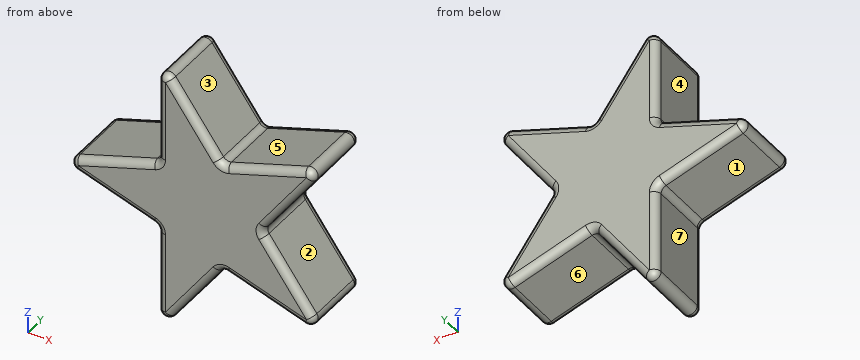
```python
from build123d import *

# Parameters (mm, degrees)
F1_DEPTH = 50.8
F2_F1_R  = 5.08
F2_F2_R  = 5.08


with BuildPart() as f1:
    # F0 (on Front) → F1 (new body)
    with BuildSketch(Plane.XZ):
        Polygon((44.7892362247, -61.6470949714), (0, 0), (44.7892362247, 61.6470949714), (-27.681270317, 38.1), (-72.4705065417, 99.7470949714), (-72.4705065417, 23.5470949714), (-144.9410130834, 0), (-72.4705065417, -23.5470949714), (-72.4705065417, -99.7470949714), (-27.681270317, -38.1), align=None)
    extrude(amount=-F1_DEPTH)

    # F2: fillet of radius 5.08 on 21 edges, made by hand

    # F2_f1
    f2_f1_edges = [f1.edges().sort_by_distance(p)[0] for p in [
        (-27.681270317, 25.4, -38.1),
        (-72.4705065417, 25.4, -23.5470949714),
        (-72.4705065417, 25.4, 23.5470949714),
        (-27.681270317, 25.4, 38.1),
        (0, 25.4, 0),
    ]]
    fillet(f2_f1_edges, radius=F2_F1_R)

    # F2_f2
    f2_f2_edges = [f1.edges().sort_by_distance(p)[0] for p in [
        (-72.4705065417, 25.4, 99.7470949714),
        (-144.9410130834, 25.4, 0),
        (44.7892362247, 25.4, 61.6470949714),
        (44.7892362247, 25.4, -61.6470949714),
        (-72.4705065417, 25.4, -99.7470949714),
        (-72.4705065417, 50.8, -63.4925129925),
        (-51.1605979265, 50.8, -70.4165220265),
        (10.3090797881, 50.8, -50.4438130159),
        (-110.4608566468, 50.8, 11.2032819554),
        (-51.1605979265, 50.8, 70.4165220265),
        (23.4793276095, 50.8, 32.3165220265),
        (23.4793276095, 0, 32.3165220265),
        (10.3090797881, 0, 50.4438130159),
        (-72.4705065417, 0, 63.4925129925),
        (-110.4608566468, 0, -11.2032819554),
        (-51.1605979265, 0, -70.4165220265),
        (-27.3106893113, 0, -39.2405310605),
        (-73.4407002103, 0, -24.251981932),
        (-73.4407002103, 0, 24.251981932),
        (-27.3106893113, 0, 39.2405310605),
        (1.1992253257, 0, 0),
        (1.1992253257, 50.8, 0),
        (-27.3106893113, 50.8, 39.2405310605),
        (-73.4407002103, 50.8, 24.251981932),
        (-27.3106893113, 50.8, -39.2405310605),
        (-73.4407002103, 50.8, -24.251981932),
    ]]
    fillet(f2_f2_edges, radius=F2_F2_R)


solid = f1.part
```
The listing builds one solid part. Answer for the finished solid, in the listing's coordinates (mm). Face numbers are marked on the shaded views. A direction names the side the tool comes from. Give positions to 0.01 mm unless a question says otherwise; leave off trailing zeros. Loops run counter-clockwise (first coordinate to the right, second up) from the corner with the lowest first, then second, coordinate; pieces in that order, holes last. Notation, with made-up numbers: (-25, 50.5) - (-13, 50.5) arc R14 ccw to (-13, 74.5) - close; hole circle Ø3 at (-39, 8). An arc over 180 degrees is marked (long way). Return JSON: item names as keys, results as strings. Group by question number.
1. Given pin 1 Ø1 at (y, z) = (38, -60) entering from -X; pin 2 Ø3 at (x, y) = (-100.5, 35.5) entering from -Z; pin 3 Ø4 at (x, y) = (-86, 30) entering from +Z, each flat-ended and moving along its own axis, determine where each tip first touches the part or whether it passes through.
2. Which of the six approach directions +Z, -Z, +X, -X, +Y, -Y give full straight-line access (tool end or side, diameter ignored) to the marked faces 4, 5, 6 and 7?
3. Determine the mould class of the marked faces 1, 2 and 3 for opening direction X: pulls with the +X half, pulls with the -X half, needs draft (parallel to the pull), parting line crosses it, or undercut.
4. Find section A-A (y = 33.5). Write down the section's boundary in (x, z).
5. Straight lines are drawn through the part: line 1 (Z direction, x = 4.5, y = 9); line 2 (Z direction, x = 14.5, y = 39); line 3 (Y direction, x = -67.5, z = 65). For each, find the intervals that lie inside material, in ascending order. Write a range as [from, to].
Verdict:
{
 "1": {"pin 1": "stops at x = -72.47", "pin 2": "stops at z = -14.93", "pin 3": "stops at z = 19.8"},
 "2": {"face 4": "+Z, -X, +Y, -Y", "face 5": "+Z, +Y, -Y", "face 6": "-Z, +Y, -Y", "face 7": "-Z, -X, +Y, -Y"},
 "3": {"face 1": "pulls with the -X half", "face 2": "pulls with the +X half", "face 3": "undercut"},
 "4": {"outline": "(-130.07, -4.83) - (-75.98, -22.41) arc R5.08 cw to (-72.47, -27.24) - (-72.47, -84.11) arc R5.08 ccw to (-63.28, -87.1) - (-29.85, -41.09) arc R5.08 cw to (-24.17, -39.24) - (29.92, -56.82) arc R5.08 ccw to (35.6, -49) - (2.17, -2.99) arc R5.08 cw to (2.17, 2.99) - (35.6, 49) arc R5.08 ccw to (29.92, 56.82) - (-24.17, 39.24) arc R5.08 cw to (-29.85, 41.09) - (-63.28, 87.1) arc R5.08 ccw to (-72.47, 84.11) - (-72.47, 27.24) arc R5.08 cw to (-75.98, 22.41) - (-130.07, 4.83) arc R5.08 ccw to start"},
 "5": {"line 1": "z = [-48.56, -6.19], [6.19, 48.56]", "line 2": "z = [-51.81, -19.96], [19.96, 51.81]", "line 3": "y = [0, 50.8]"}
}
